```python
from build123d import *

# Parameters (mm, degrees)
F0_W     = 38.1
F0_H     = 222.25
F1_DEPTH = 88.9
F0_H_2   = 88.9
F2_DEPTH = 50.8


with BuildPart() as f1:
    # F0 (on Top) → F1 (new body)
    with BuildSketch(Plane.XY):
        with Locations((0, -44.45)):
            Rectangle(F0_W, F0_H)
    extrude(amount=-F1_DEPTH)

    # F0 (on Top) → F2 (join)
    with BuildSketch(Plane.XY):
        with Locations((0, 111.125)):
            Rectangle(F0_W, F0_H_2)
    extrude(amount=-F2_DEPTH)


solid = f1.part
```
Could you check a few things on this model? Use its own coordinates, in mm. A direction names the side the tool comes from. Round coordinates to 2 decimals unless told otherwise and drop trailing zeros. Loops run counter-clockwise (first coordinate to the right, second up) from the corner with the lowest first, then second, coordinate; pieces in that order, holes last. Notation, with made-up numbers: (28.5, -34.75) -> (85.5, -34.75) arc R29 ccw to (85.5, 4.25) -> close; hole circle Ø8 at (51.5, -11.5). An arc over 180 degrees is marked (long way). Put each result on its own line as item: value.
Q1. Which directions (+Z, -Z, +X, -X, +Y, -Y) give clear straight access to the entire face, cutting with the end or side of a thin tool? Please do faces 1 (the flat face through (0, 155.575, -25)), 2 (the flat face through (0, 112, -50.8)).
Checks:
face 1: +Z, -Z, +X, -X, +Y
face 2: -Z, +X, -X, +Y
Q2. Please list where these lines run through material, in increasing order: line 1 (Y direction, x = -3.5, z = -59.5) (3 decimals); line 2 (Z direction, x = -14, y = 70). Write a range as from..to.
Checks:
line 1: -155.575..66.675
line 2: -50.8..0
Q3. I want a section at A-A on x = 4.5. Write out the boundary of the cut face in (y, z) (3 decimals), and give its area (3 significant figures).
Checks:
outline: (-155.575, -88.9) -> (66.675, -88.9) -> (66.675, -50.8) -> (155.575, -50.8) -> (155.575, 0) -> (-155.575, 0) -> close
area: 24,300 mm2
Q4. For pin 1 Ø11.5 at (x, z) = (2, -76) entering from +Y (3 decimals); pin 2 Ø3 at (x, y) = (12, 60.5) entering from +Z; pin 3 Ø11.5 at (x, y) = (-5.5, 89.5) entering from -Z, each with a flat end and sliding along its axis, tell me the tip position at first contact or that it passes through.
Checks:
pin 1: y = 66.675
pin 2: z = 0
pin 3: z = -50.8
Q5. I want a section at B-B on z = -80. Write out the boundary of the cut face in (x, y) (3 decimals), and give its area (3 significant figures).
Checks:
outline: (-19.05, -155.575) -> (19.05, -155.575) -> (19.05, 66.675) -> (-19.05, 66.675) -> close
area: 8,470 mm2
Q6. I want a section at C-C on y = 132. Write out the boundary of the cut face in (x, z), and give its area (3 significant figures).
Checks:
outline: (-19.05, -50.8) -> (19.05, -50.8) -> (19.05, 0) -> (-19.05, 0) -> close
area: 1,940 mm2
